The listing builds one solid part. Answer for the finished solid, in the listing's coordinates (mm). Face numbers are marked on the shaded views. A direction names the side the tool comes from. Coordinates: 2 decimals unless noted, no trailing zeros. Loops run counter-clockwise (first coordinate to the right, second up) from the corner with the lowest first, then second, coordinate; pieces in that order, holes last. Notation, with made-up numbers: M 73,-30.75 L 116,-30.75 A5 ccw 116,-22.75 Z; hole C 25,45.5 d4. An arc over 180 degrees is marked long. Answer in a Markdown table with one row per item. Add a question column.
from build123d import *

# Parameters (mm, degrees)
SKETCH1_R           = 70
BOSS_EXTRUDE1_DEPTH = 35
SHELL6_T            = -10
BOSS_EXTRUDE3_DEPTH = 25
SHELL13_T           = -1
CIRPATTERN6_COUNT   = 4
CIRPATTERN7_DEPTH   = 26
SKETCH2_R           = 35
CUT_EXTRUDE5_DEPTH  = 7
SKETCH6_R           = 10.5
CUT_EXTRUDE6_DEPTH  = 7


# Read off the part's stored shape, not the designer's step: CirPattern7
with BuildPart() as part:
    # Sketch1 → Boss-Extrude1 (new body)
    with BuildSketch(Plane(origin=(0, 0, 0), x_dir=(1, 0, 0), z_dir=(0, 1, 0))):
        with Locations(Location((0, 0, 0), (0, 0, 270))):
            Circle(SKETCH1_R)
    extrude(amount=BOSS_EXTRUDE1_DEPTH)

    # Shell6
    shell6_openings = [part.faces().sort_by_distance(p)[0] for p in [
        (0, 0, 0),
    ]]
    offset(amount=SHELL6_T, openings=shell6_openings, kind=Kind.INTERSECTION)

    # Sketch5 → Boss-Extrude3 (add, through all)
    with BuildSketch(Plane.XZ.offset(-25)):
        Polygon((-55, 4.907477288), (-59.25, 2.453738644), (-59.25, -2.453738644), (-55, -4.907477288), (-50.75, -2.453738644), (-50.75, 2.453738644), align=None)
    boss_extrude3 = extrude(amount=BOSS_EXTRUDE3_DEPTH)

    # Shell13
    shell13_openings = [part.faces().sort_by_distance(p)[0] for p in [
        (-55, 0, 0),
    ]]
    offset(amount=SHELL13_T, openings=shell13_openings, kind=Kind.INTERSECTION)

    # CirPattern6: Boss-Extrude3 ×4 about axis
    cirpattern6_axis = Axis((0, 0, 0), (0, 1, 0))
    for i in range(1, CIRPATTERN6_COUNT):
        add(boss_extrude3.rotate(cirpattern6_axis, i * 360 / CIRPATTERN6_COUNT))

    # CirPattern7 outline → CirPattern7 (cut)
    with BuildSketch(Plane(origin=(0, 0, 0), x_dir=(1, 0, 0), z_dir=(0, 1, 0))):
        Polygon((-1.876388375, 51.75), (1.876388375, 51.75), (3.75277675, 55), (1.876388375, 58.25), (-1.876388375, 58.25), (-3.75277675, 55), align=None)
        Polygon((51.75, -1.876388375), (55, -3.75277675), (58.25, -1.876388375), (58.25, 1.876388375), (55, 3.75277675), (51.75, 1.876388375), align=None)
        Polygon((1.876388375, -51.75), (-1.876388375, -51.75), (-3.75277675, -55), (-1.876388375, -58.25), (1.876388375, -58.25), (3.75277675, -55), align=None)
    extrude(amount=CIRPATTERN7_DEPTH, mode=Mode.SUBTRACT)

    # Sketch2 → Cut-Extrude5 (cut)
    with BuildSketch(Plane(origin=(0, 35, 0), x_dir=(1, 0, 0), z_dir=(0, 1, 0))):
        with Locations(Location((0, 0, 0), (0, 0, 270))):
            Circle(SKETCH2_R)
    extrude(amount=-CUT_EXTRUDE5_DEPTH, mode=Mode.SUBTRACT)

    # Sketch6 → Cut-Extrude6 (cut)
    with BuildSketch(Plane(origin=(0, 26, 0), x_dir=(1, 0, 0), z_dir=(0, 1, 0))):
        with Locations(Location((0, 0, 0), (0, 0, 270))):
            Circle(SKETCH6_R)
    extrude(amount=-CUT_EXTRUDE6_DEPTH, mode=Mode.SUBTRACT)


solid = part.part
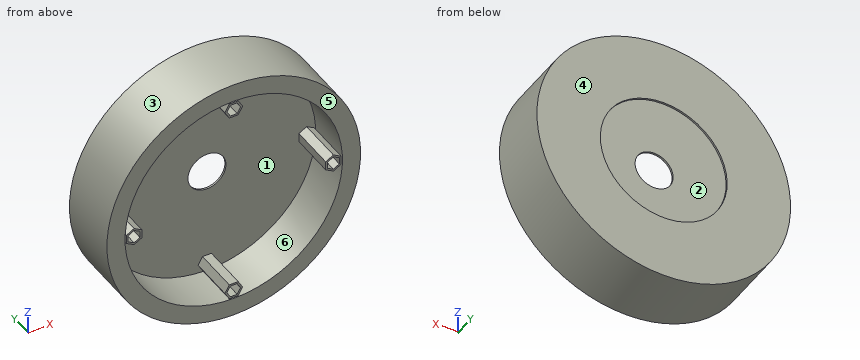
(1) A cutting plane is placed at A-A (y = 30.5). Give the vertices of the cut face in (x, z), plus the area to 3 significant figures.
(2) Straight lines are drawn through the part: line 1 (X direction, y = 25.4, z = 0); line 2 (X direction, y = 12, z = -4); line 3 (Y direction, x = 22, z = -56.5). For each, find the intervals that lie inside material, in ascending order.
(3) For the marked faces 5 and 6, determine the directions among +Z, -Z, +X, -X, +Y, -Y from which every point of the face is accessible in a straight line to the end or side of a thin tool.
(4) Each of these flat-tipped pins is pushed along its axis until it touches: pin 1 (4 mm diameter, centred on y = 10.5, z = 0.5, fed in from -X); pin 2 (2 mm diameter, centred on y = 7.5, z = 44, fed in from +X); pin 3 (10 mm diameter, centred on x = 46, y = 7, fed in from -Z); pin 4 (12.5 mm diameter, centred on x = 0, z = 0, fed in from -Y). Where does it stop, or does it pass through?
(5) The mould has two halves that part along Y. Classify the marked faces 1, 2, 3 and 4: released by +Y, released by -Y, zero draft, split by the parting line, or undercut.
(6) A cutting plane is placed at D-D (x = -20). Give the vertices of the cut face in (y, z).
(7) A cutting plane is placed at B-B (z = 0). State how many separate pieces and enclosed holes the cut face has, plus the area to 3 significant figures.
Solved:
| question | item | result |
|---|---|---|
| 1 | outline | C 0,0 d140; hole C 0,0 d138 |
| 1 | area | 437 mm² |
| 2 | line 1 | x = -70 to -69, -61 to -58.25, -51.75 to -10.5, 10.5 to 51.75, 58.25 to 61, 69 to 70 |
| 2 | line 2 | x = -69.89 to -68.88, -60.87 to -59.87, -56.57 to -53.43, 53.43 to 56.57, 59.87 to 60.87, 68.88 to 69.89 |
| 2 | line 3 | y = 0 to 26, 34 to 35 |
| 3 | face 5 | +Z, -Z, +X, -X, -Y |
| 3 | face 6 | -Y |
| 4 | pin 1 | stops at x = -70 |
| 4 | pin 2 | stops at x = 55.24 |
| 4 | pin 3 | stops at z = -56.74 |
| 4 | pin 4 | passes through |
| 5 | face 1 | released by -Y |
| 5 | face 2 | undercut |
| 5 | face 3 | zero draft |
| 5 | face 4 | released by +Y |
| 6 | outline | M 0,-67.08 L 35,-67.08 L 35,-28.72 L 34,-28.72 L 34,-66.04 L 1,-66.04 L 1,-57.63 L 26,-57.63 L 26,57.63 L 1,57.63 L 1,66.04 L 34,66.04 L 34,28.72 L 35,28.72 L 35,67.08 L 0,67.08 L 0,56.57 L 25,56.57 L 25,-56.57 L 0,-56.57 Z |
| 7 | separate pieces | 4 |
| 7 | enclosed holes | 0 |
| 7 | area | 392 mm² |
